For this review, take the finished solid that the model builds, in its own axes (mm). Face numbers are marked on the shaded views. A direction names the side the tool comes from. Round coordinates to 2 decimals unless told otherwise and drop trailing zeros. Loops run counter-clockwise (first coordinate to the right, second up) from the corner with the lowest first, then second, coordinate; pieces in that order, holes last. Notation, with made-up numbers: (67.5, -13.75) -> (83.5, -13.75) arc R38 cw to (83.5, 24.25) -> close; hole circle Ø8 at (22.25, 29.25). An arc over 180 degrees is marked (long way). One line per question, with ' | ' between items. Start each with the question number.
1. Wall thickness on line 1 along X through (y, z) = (-7.5, 4); line 2 along X through (y, z) = (-3, 3.25); line 3 along X through (y, z) = (3, 2.75): over which ranges is each line inside the solid? List them lowest first.
2. For pin 1 Ø3 at (y, z) = (8, 1) entering from -X, flat-tipped, find the tip position at first contact; note if it passes through.
3. Consider section D-D (y = 6.75). Write out the cut boundary in (x, z) (3 decimals).
4. Consider section B-B (z = 2). Write out the cut boundary in (x, y), and give its area (3 significant figures).
5. Draft analysis for pull direction X (two halves, no side actions). For the marked faces 6, 7, 8 and 9, state which applies: pulls with the +X half, pulls with the -X half, needs draft (parallel to the pull), parting line crosses it, or undercut.
6. Consider section C-C (x = -7.5). Write out the cut boundary in (y, z).
7. For the marked faces 1, 2, 3, 4 and 5, list the 3-axis set-ups (+Z, -Z, +X, -X, +Y, -Y) from which the entire face can be reached by the end or side of a thin tool; tool diameter is ignored.
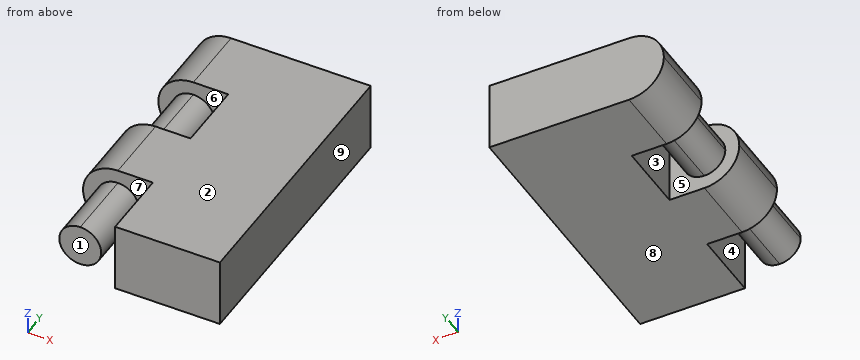
```python
from build123d import *

# Parameters (mm, degrees)
F0_W     = 12.7
F0_H     = 25.4
F1_DEPTH = 6.35
F3_DEPTH = 25.4
F4_DEPTH = 25.4
F5_W     = 3.1755
F5_H     = 6.35
F5_W_2   = 3.1745
F6_DEPTH = 25.4
F7_DEPTH = 25.4


with BuildPart() as f1:
    # F0 (on Top) → F1 (new body)
    with BuildSketch(Plane.XY):
        Rectangle(F0_W, F0_H)
    extrude(amount=F1_DEPTH)

    # F2 (on face) → F3 (join)
    with BuildSketch(Plane(origin=(0, 12.7, 0), x_dir=(-1, 0, 0), z_dir=(0, 1, 0))):
        with BuildLine():
            Line((6.35, 5.08), (6.35, 6.35))
            ThreePointArc((6.35, 6.35), (3.175, 3.175), (6.35, 0))
            Line((6.35, 0), (6.35, 1.27))
            ThreePointArc((6.35, 1.27), (4.445, 3.175), (6.35, 5.08))
        make_face()
        with BuildLine():
            ThreePointArc((-6.35, 0), (-4.104936, 0.929936), (-3.175, 3.175))
            ThreePointArc((-3.175, 3.175), (-4.104936, 5.420064), (-6.35, 6.35))
            Line((-6.35, 6.35), (-6.35, 5.08))
            ThreePointArc((-6.35, 5.08), (-5.002962, 4.522038), (-4.445, 3.175))
            ThreePointArc((-4.445, 3.175), (-5.002962, 1.827962), (-6.35, 1.27))
            Line((-6.35, 1.27), (-6.35, 0))
        make_face()
        with BuildLine():
            ThreePointArc((9.525, 3.175), (8.595064, 5.420064), (6.35, 6.35))
            Line((6.35, 6.35), (6.35, 5.08))
            ThreePointArc((6.35, 5.08), (7.697038, 4.522038), (8.255, 3.175))
            ThreePointArc((8.255, 3.175), (7.697038, 1.827962), (6.35, 1.27))
            Line((6.35, 1.27), (6.35, 0))
            ThreePointArc((6.35, 0), (8.595064, 0.929936), (9.525, 3.175))
        make_face()
        with BuildLine():
            ThreePointArc((-4.445, 3.175), (-5.002962, 4.522038), (-6.35, 5.08))
            Line((-6.35, 5.08), (-6.35, 1.27))
            ThreePointArc((-6.35, 1.27), (-5.002962, 1.827962), (-4.445, 3.175))
        make_face()
    extrude(amount=-F3_DEPTH)

    # F2 (on face) → F4 (cut)
    with BuildSketch(Plane(origin=(0, 12.7, 0), x_dir=(-1, 0, 0), z_dir=(0, 1, 0))):
        with BuildLine():
            Line((-6.35, 1.27), (-6.35, 5.08))
            ThreePointArc((-6.35, 5.08), (-8.255, 3.175), (-6.35, 1.27))
        make_face()
        with BuildLine():
            ThreePointArc((8.255, 3.175), (7.697038, 4.522038), (6.35, 5.08))
            Line((6.35, 5.08), (6.35, 1.27))
            ThreePointArc((6.35, 1.27), (7.697038, 1.827962), (8.255, 3.175))
        make_face()
    extrude(amount=-F4_DEPTH, mode=Mode.SUBTRACT)

    # F5 (on face) → F6 (cut)
    with BuildSketch(Plane(origin=(0, 0, 0), x_dir=(1, 0, 0), z_dir=(0, 0, -1))):
        with Locations((-7.93775, 9.525)):
            Rectangle(F5_W, F5_H)
        with Locations((-7.93775, -3.175)):
            Rectangle(F5_W, F5_H)
        with Locations((-4.76275, 9.525)):
            Rectangle(F5_W_2, F5_H)
        with Locations((-4.76275, -3.175)):
            Rectangle(F5_W_2, F5_H)
    extrude(amount=-F6_DEPTH, mode=Mode.SUBTRACT)

    # F2 (on face) → F7 (join)
    with BuildSketch(Plane(origin=(0, 12.7, 0), x_dir=(-1, 0, 0), z_dir=(0, 1, 0))):
        with BuildLine():
            ThreePointArc((8.255, 3.175), (7.697038, 4.522038), (6.35, 5.08))
            Line((6.35, 5.08), (6.35, 1.27))
            ThreePointArc((6.35, 1.27), (7.697038, 1.827962), (8.255, 3.175))
        make_face()
        with BuildLine():
            Line((6.35, 1.27), (6.35, 5.08))
            ThreePointArc((6.35, 5.08), (4.445, 3.175), (6.35, 1.27))
        make_face()
    extrude(amount=-F7_DEPTH)


solid = f1.part
```
Answer block:
1) line 1: x = -8.07 to -4.63, -3.18 to 6.35 | line 2: x = -9.52 to 6.35 | line 3: x = -8.21 to -4.49, -3.18 to 6.35
2) pin 1: stops at x = -9.45
3) outline: (-6.35, 0) -> (6.35, 0) -> (6.35, 6.35) -> (-6.35, 6.35) arc R3.175 ccw to start
4) outline: (-9.3, -6.35) -> (-7.85, -6.35) -> (-7.85, -12.7) -> (-4.85, -12.7) -> (-4.85, -6.35) -> (-3.18, -6.35) -> (-3.18, -12.7) -> (6.35, -12.7) -> (6.35, 12.7) -> (-9.3, 12.7) -> (-9.3, 6.35) -> (-7.85, 6.35) -> (-7.85, 0) -> (-9.3, 0) -> close; hole (-4.85, 0) -> (-3.18, 0) -> (-3.18, 6.35) -> (-4.85, 6.35) -> close | area: 358 mm2
5) face 6: undercut | face 7: undercut | face 8: needs draft | face 9: pulls with the +X half
6) outline: (-12.7, 1.66) -> (-6.35, 1.66) -> (-6.35, 0.22) -> (0, 0.22) -> (0, 1.66) -> (6.35, 1.66) -> (6.35, 0.22) -> (12.7, 0.22) -> (12.7, 6.13) -> (6.35, 6.13) -> (6.35, 4.69) -> (0, 4.69) -> (0, 6.13) -> (-6.35, 6.13) -> (-6.35, 4.69) -> (-12.7, 4.69) -> close
7) face 1: +Z, -Z, +X, -X, -Y | face 2: +Z, +X, -X, +Y, -Y | face 3: +Z, -Z | face 4: +Z, -Z, -Y | face 5: none
